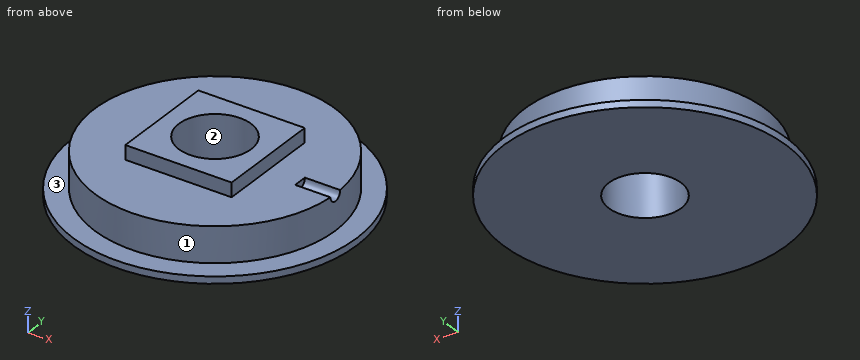
Autodesk Inventor part; units mm, degrees
ref_plane "Arbeitsebene2" through (17, 0, 0) normal (1, 0, 0) x (0, 1, 0)
ref_plane "XZ Plane" through (0, 0, 0) normal (0, 1, 0) x (-1, 0, 0)
ref_plane "XY Plane" through (0, 0, 0) normal (0, 0, 1) x (1, 0, 0)
sketch "Skizze1" plane through (0, 0, 0) normal (0, 0, 1) x (1, 0, 0)
  circle A0 centre (0, 0) radius 20
  dimension "d0" = 40
extrude "Extrusion1" add sketch "Skizze1" along normal blind 1
sketch "Skizze2" plane through (0, 0, 1) normal (0, 0, 1) x (1, 0, 0)
  circle A0 centre (0, 0) radius 20
  circle A1 centre (0, 0) radius 17
  dimension "d3" = 34
extrude "Extrusion2" add sketch "Skizze2" along normal blind 10 contours A1
sketch "Skizze3" plane through (0, 0, 11) normal (0, 0, 1) x (1, 0, 0)
  circle A0 centre (0, 0) radius 17
  circle A1 centre (0, 0) radius 20
  dimension "d6" = 40
extrude "Extrusion3" add sketch "Skizze3" along normal blind 1 contours A0 | A1
sketch "Skizze6" plane through (0, 0, 12) normal (0, 0, 1) x (1, 0, 0)
  circle A0 centre (0, 0) radius 20
  circle A1 centre (0, 0) radius 5.1
  dimension "d16" = 10.2
extrude "Extrusion6" cut sketch "Skizze6" against normal through all contours A1
sketch "Skizze7" plane through (0, 0, 0) normal (0, 1, 0) x (-1, 0, 0)
  line L0 (17, 1) -> (17, 11)
  line L1 (-17, 1) -> (-17, 11)
  line L2 (20, 0) -> (-20, 0)
  line L3 (20, 0) -> (20, 1)
  line L4 (20, 1) -> (-20, 1)
  line L5 (-17, 1) -> (-17, 11)
  line L6 (20, 0) -> (-20, 0)
  line L7 (-20, 0) -> (-20, 6)
  line L8 (-20, 6) -> (20, 6)
  line L9 (20, 6) -> (20, 0)
  line L10 (20, 12) -> (-20, 12)
  point P0 (0, 0)
  dimension "d19" = 6
  dimension "d20" = 12
extrude "Extrusion7" cut sketch "Skizze7" along normal through all both and the other way through all keep common part
ref_plane "Arbeitsebene2" through (17, 0, 0) normal (1, 0, 0) x (0, 1, 0)
sketch "Skizze9" plane through (17, 0, 0) normal (1, 0, 0) x (0, 1, 0)
  line L0 (17, 6) -> (-17, 6)
  circle A0 centre (0, 6) radius 1
  point P0 (0, 0)
  point P1 (-1, 6)
  point P2 (1, 6)
  dimension "d24" = 2
extrude "Extrusion8" cut sketch "Skizze9" against normal blind 5 contours A0 L0 picked at (0.0402, 5.6691)
sketch "Skizze10" plane through (12, 1, 6) normal (0, 0, 1) x (1, 0, 0)
  circle A0 centre (-12, -1) radius 5.1
  line L0 (-19.5, 6.5) -> (-4.5, 6.5)
  line L1 (-4.5, 6.5) -> (-4.5, -8.5)
  line L2 (-4.5, -8.5) -> (-19.5, -8.5)
  line L3 (-19.5, -8.5) -> (-19.5, 6.5)
  line L4 (-19.5, 6.5) -> (-4.5, -8.5) construction
  line L5 (-4.5, 6.5) -> (-19.5, -8.5) construction
  dimension "d27" = 15
  dimension "d28" = 15
extrude "Extrusion9" add sketch "Skizze10" along normal blind 2
equation "\"d19\" = 0.5 * d20"
equation "\"d28\" = d27"
properties part number "Motorstange_version2a"
Work out the finished part from the listing and answer in its coordinate system (mm). Face numbers are marked on the shaded views. Coordinates: 2 decimals unless noted, no trailing zeros. Write each loop counter-clockwise with the first axis right and the second up, starting at its lowest first coordinate (ties: lowest second). Pieces come first, ordered by that corner, then holes.
Q1. Find the intervals of material crossed by line 1 (Y direction, x = 0, z = 4.5); line 2 (Z direction, x = 16.5, y = -9.5); line 3 (Y direction, x = 4, z = 4.75), in increasing order.
Q2. A cutting plane is placed at D-D, the plane y = 14. Give the vertices of the cut face in (x, z).
Q3. A cutting plane is placed at A-A, the plane x = 0. Give the vertices of the cut face in (y, z).
Q4. Each of these flat-tipped pins is pushed along its axis until it touches: pin 1 Ø1 at (y, z) = (2.5, 7) entering from +X; pin 2 Ø8 at (x, y) = (0, 0) entering from +Z; pin 3 Ø1 at (y, z) = (4, 7) entering from -X; pin 4 Ø3 at (x, y) = (-2.5, -11) entering from +Z. Where does it stop, or does it pass through?
Q5. A cutting plane is placed at B-B, the plane y = -3.5. Give the vertices of the cut face in (x, z), then the cut area to 3 significant figures.
Q6. Determine the mould class of the marked faces 1, 2 and 3 for opening direction X: released by +X, released by -X, zero draft, split by the parting line, or undercut.
Q7. A cutting plane is placed at C-C, the plane z = 6.75. Give the vertices of the cut face in (x, y), then the cut area to 3 significant figures.
Findings below:
1. line 1: y = -17 to -5.1, 5.1 to 17
1. line 2: z = 0 to 1
1. line 3: y = -16.52 to -3.16, 3.16 to 16.52
2. outline: (-14.28, 0) - (14.28, 0) - (14.28, 1) - (9.64, 1) - (9.64, 6) - (-9.64, 6) - (-9.64, 1) - (-14.28, 1) - close
3. outline: (-20, 0) - (-5.1, 0) - (-5.1, 8) - (-7.5, 8) - (-7.5, 6) - (-17, 6) - (-17, 1) - (-20, 1) - close; (5.1, 0) - (20, 0) - (20, 1) - (17, 1) - (17, 6) - (7.5, 6) - (7.5, 8) - (5.1, 8) - close
4. pin 1: stops at x = 7.5
4. pin 2: passes through
4. pin 3: stops at x = -7.5
4. pin 4: stops at z = 6
5. outline: (-19.69, 0) - (-3.71, 0) - (-3.71, 8) - (-7.5, 8) - (-7.5, 6) - (-16.64, 6) - (-16.64, 1) - (-19.69, 1) - close; (3.71, 0) - (19.69, 0) - (19.69, 1) - (16.64, 1) - (16.64, 6) - (7.5, 6) - (7.5, 8) - (3.71, 8) - close
5. area: 176 mm2
6. face 1: split by the parting line
6. face 2: undercut
6. face 3: zero draft
7. outline: (-7.5, -7.5) - (7.5, -7.5) - (7.5, 7.5) - (-7.5, 7.5) - close; hole circle Ø10.2 at (0, 0)
7. area: 143 mm2
